```python
from build123d import *

# Parameters (mm, degrees)
SKETCH1_R           = 2.5
BOSS_EXTRUDE1_DEPTH = 195


with BuildPart() as part:
    # Sketch1 → Boss-Extrude1 (new body)
    with BuildSketch(Plane.XY):
        with BuildLine():
            Line((9.573137603, 3.497470387), (10, 3.497470387))
            Line((10, 3.497470387), (10, 8.397470387))
            ThreePointArc((10, 8.397470387), (9.598622578, 9.525052949), (8.5, 10))
            Line((8.5, 10), (3.6, 10))
            Line((3.6, 10), (3.6, 9.479132912))
            Line((3.6, 9.479132912), (3.075, 9.479132912))
            Line((3.075, 9.479132912), (3.075, 8.2))
            Line((3.075, 8.2), (5.304654122, 8.2))
            Line((5.304654122, 8.2), (5.304654122, 6.8))
            Line((5.304654122, 6.8), (2.404654122, 3.9))
            Line((2.404654122, 3.9), (-2.404654122, 3.9))
            Line((-2.404654122, 3.9), (-5.304654122, 6.94037733))
            Line((-5.304654122, 6.94037733), (-5.304654122, 8.2))
            Line((-5.304654122, 8.2), (-3.075, 8.2))
            Line((-3.075, 8.2), (-3.075, 9.565763355))
            Line((-3.075, 9.565763355), (-3.497470387, 9.573137603))
            Line((-3.497470387, 9.573137603), (-3.497470387, 10))
            Line((-3.497470387, 10), (-8.397470387, 10))
            ThreePointArc((-8.397470387, 10), (-9.525052949, 9.598622578), (-10, 8.5))
            Line((-10, 8.5), (-10, 3.6))
            Line((-10, 3.6), (-9.479132912, 3.6))
            Line((-9.479132912, 3.6), (-9.479132912, 3.075))
            Line((-9.479132912, 3.075), (-8.2, 3.075))
            Line((-8.2, 3.075), (-8.2, 5.304654122))
            Line((-8.2, 5.304654122), (-6.8, 5.304654122))
            Line((-6.8, 5.304654122), (-3.9, 2.404654122))
            Line((-3.9, 2.404654122), (-3.9, -2.404654122))
            Line((-3.9, -2.404654122), (-6.94037733, -5.304654122))
            Line((-6.94037733, -5.304654122), (-8.2, -5.304654122))
            Line((-8.2, -5.304654122), (-8.2, -3.075))
            Line((-8.2, -3.075), (-9.565763355, -3.075))
            Line((-9.565763355, -3.075), (-9.573137603, -3.497470387))
            Line((-9.573137603, -3.497470387), (-10, -3.497470387))
            Line((-10, -3.497470387), (-10, -8.397470387))
            ThreePointArc((-10, -8.397470387), (-9.598622578, -9.525052949), (-8.5, -10))
            Line((-8.5, -10), (-3.6, -10))
            Line((-3.6, -10), (-3.6, -9.479132912))
            Line((-3.6, -9.479132912), (-3.075, -9.479132912))
            Line((-3.075, -9.479132912), (-3.075, -8.2))
            Line((-3.075, -8.2), (-5.304654122, -8.2))
            Line((-5.304654122, -8.2), (-5.304654122, -6.8))
            Line((-5.304654122, -6.8), (-2.404654122, -3.9))
            Line((-2.404654122, -3.9), (2.404654122, -3.9))
            Line((2.404654122, -3.9), (5.304654122, -6.94037733))
            Line((5.304654122, -6.94037733), (5.304654122, -8.2))
            Line((5.304654122, -8.2), (3.075, -8.2))
            Line((3.075, -8.2), (3.075, -9.565763355))
            Line((3.075, -9.565763355), (3.497470387, -9.573137603))
            Line((3.497470387, -9.573137603), (3.497470387, -10))
            Line((3.497470387, -10), (8.397470387, -10))
            ThreePointArc((8.397470387, -10), (9.525052949, -9.598622578), (10, -8.5))
            Line((10, -8.5), (10, -3.6))
            Line((10, -3.6), (9.479132912, -3.6))
            Line((9.479132912, -3.6), (9.479132912, -3.075))
            Line((9.479132912, -3.075), (8.2, -3.075))
            Line((8.2, -3.075), (8.2, -5.304654122))
            Line((8.2, -5.304654122), (6.8, -5.304654122))
            Line((6.8, -5.304654122), (3.9, -2.404654122))
            Line((3.9, -2.404654122), (3.9, 2.404654122))
            Line((3.9, 2.404654122), (6.94037733, 5.304654122))
            Line((6.94037733, 5.304654122), (8.2, 5.304654122))
            Line((8.2, 5.304654122), (8.2, 3.075))
            Line((8.2, 3.075), (9.565763355, 3.075))
            Line((9.565763355, 3.075), (9.573137603, 3.497470387))
        make_face()
        Circle(SKETCH1_R, mode=Mode.SUBTRACT)
    extrude(amount=BOSS_EXTRUDE1_DEPTH)


solid = part.part
```
Part model, mm, in its own coordinate system. A direction names the side the tool comes from. Round coordinates to 2 decimals unless told otherwise and drop trailing zeros. Write each loop counter-clockwise with the first axis right and the second up, starting at its lowest first coordinate (ties: lowest second). Pieces come first, ordered by that corner, then holes.
Item 1: Which spindle directions (+Z, -Z, +X, -X, +Y, -Y) get a long thin tool onto all of the face, cutting with end or side? Do faces 1 (the flat face through (-2, 2, 195)), 2 (the flat face through (-5.399, -3.834, 96.135)), 3 (the flat face through (0, -3.9, 96)). Say none if no direction does.
Results:
face 1: +Z, +X, -X, +Y, -Y
face 2: +Z, -Z
face 3: +Z, -Z, -Y
Item 2: Cut at A-A, the plane y = 0. Give the cut face in (x, z).
Results:
outline: (-3.9, 0) - (-2.5, 0) - (-2.5, 195) - (-3.9, 195) - close; (2.5, 0) - (3.9, 0) - (3.9, 195) - (2.5, 195) - close
Item 3: Probe L1, parallel to Y at x = -7.25, z = 115; L2, parallel to Y at x = -5.25, z = 118. List the from-to ranges inside material, lowest first.
Results:
L1: y = -10 to -5.3, 5.3 to 10
L2: y = -10 to -8.2, -6.75 to -3.69, 3.75 to 6.88, 8.2 to 10
Item 4: Two-plate mould, pull along X, no slides. Class faces 4 (the flat face through (6, 10, 96)), 5 (the flat face through (-3.9, 0, 96)), 6 (the flat face through (0, 3.9, 96)), 7 (the flat face through (5.399, 3.834, 96.135)): +X half, -X half, draft (parallel to the pull), parting line (faces both ways), or undercut.
Results:
face 4: draft
face 5: -X half
face 6: undercut
face 7: undercut
Item 5: Drop flat-ended pins along their axis: pin 1 Ø0.6 at (x, z) = (-3.5, 113) entering from -Y; pin 2 Ø1.1 at (y, z) = (4, 49.5) entering from +X; pin 3 Ø2 at (x, y) = (4.5, 7.5) entering from -Z; pin 4 Ø6 at (y, z) = (-3, 172.5) entering from -X. Give the stop position or say it passes through.
Results:
pin 1: stops at y = -10
pin 2: stops at x = 10
pin 3: stops at z = 0
pin 4: stops at x = -10
